Could you check a few things on this model? Use its own coordinates, in mm. A direction names the side the tool comes from. Give positions to 0.01 mm unless a question says otherwise; leave off trailing zeros. Write each loop counter-clockwise with the first axis right and the second up, starting at its lowest first coordinate (ties: lowest second). Pieces come first, ordered by that corner, then holes. Notation, with made-up numbers: M 11.25,63 L 60.25,63 A7 ccw 60.25,74 Z; hole C 63,79 d5. An arc over 180 degrees is marked long. Answer as CSV lines item,"result". Start each with the question number.
Autodesk Inventor part; units mm, degrees
ref_plane "作業平面1" through (0, 0, 29) normal (0, 0, 1) x (1, 0, 0)
ref_plane "YZ Plane" through (0, 0, 0) normal (1, 0, 0) x (0, 1, 0)
ref_plane "XZ Plane" through (0, 0, 0) normal (0, 1, 0) x (-1, 0, 0)
sketch "スケッチ1" plane through (0, 0, 0) normal (0, 0, 1) x (1, 0, 0)
  circle A0 centre (0, 0) radius 1.5
  circle A1 centre (0, 0) radius 3
  dimension "d0" = 3
  dimension "d1" = 6
extrude "押し出し1" add sketch "スケッチ1" along normal blind 35
ref_plane "作業平面1" through (0, 0, 29) normal (0, 0, 1) x (1, 0, 0)
sketch "スケッチ3" plane through (0, 0, 29) normal (0, 0, 1) x (1, 0, 0)
  circle A0 centre (0, 0) radius 1.5
extrude "押し出し3" add sketch "スケッチ3" against normal blind 23
sketch "スケッチ4" plane through (0, 0, 0) normal (0, 0, -1) x (-1, 0, 0)
  circle A0 centre (0, 0) radius 3
  circle A1 centre (0, 0) radius 1.5
  circle A2 centre (0, 0) radius 3
  circle A3 centre (0, 0) radius 4
  dimension "d9" = 8
extrude "押し出し4" add sketch "スケッチ4" against normal blind 35 contours A3
sketch "スケッチ5" plane through (0, 0, 35) normal (0, 0, 1) x (1, 0, 0)
  circle A0 centre (0, 0) radius 1.5
  circle A1 centre (0, 0) radius 2
  dimension "d12" = 4
extrude "押し出し5" cut sketch "スケッチ5" against normal blind 6 contours A0 | A1
properties part number "スペーサー自作m3,35" material "アルミニウム 7075"
1. On a 3-axis mill with a long thin cutter (end or side, diameter ignored), from which of +Z, -Z, +X, -X, +Y, -Y can I reach the whole of each face in a straight line? I mean faces 5 (the flat face through (2, -1, 35)), 6 (the flat face through (0, 0, 29)), 7 (the flat face through (0, 0, 6)). Say none if no direction works.
2. Imagine slicing it at D-D, the plane y = 3.25. Please give me the cut outline in (x, z), plus the area to 3 significant figures.
3. Imagine slicing it at B-B, the plane z = 25.5. Please give me the cut outline in (x, y).
4. Imagine slicing it at C-C, the plane y = -2.75. Please give me the cut outline in (x, z), plus the area to 3 significant figures.
5. Thinking about a two-plate mould opening in X: for faces 1 (the flat face through (-2, 0, 0)), 2 (the cylindrical face through (0.867, -3.905, 17.255)), 3 (the cylindrical face through (-1.5, -0.07, 2.96)), 4 (the cylindrical face through (0, -2, 32)), which applies, pulls with the +X half, pulls with the -X half, needs draft (parallel to the pull), parting line crosses it, or undercut?
6. Please list where these lines run through material, in increasing order: line 1 (Y direction, x = 0, z = 4.05); line 2 (Y direction, x = 0, z = 32.85); line 3 (Z direction, x = -1.75, y = 0).
7. Will these pins go through, and if not, where does the flat tip stop? P1, Ø3, axis at x = -2.5, z = 14.5, coming from the +Y side; P2, Ø1.5, axis at x = 0, y = 0.5, coming from the -Z side; P3, Ø1.2, axis at x = -0.5, y = -0.5, coming from the +Z side.
8. Imagine slicing it at A-A, the plane x = 0. Please give me the cut outline in (y, z), plus the area to 3 significant figures.
Solutions:
1,face 5,"+Z, +X, -X, +Y, -Y"
1,face 6,"+Z"
1,face 7,"-Z"
2,outline,"M -2.33,0 L 2.33,0 L 2.33,35 L -2.33,35 Z"
2,area,"163 mm²"
3,outline,"C 0,0 d8"
4,outline,"M -2.9,0 L 2.9,0 L 2.9,35 L -2.9,35 Z"
4,area,"203 mm²"
5,face 1,"needs draft"
5,face 2,"parting line crosses it"
5,face 3,"undercut"
5,face 4,"undercut"
6,line 1,"-4 to -1.5, 1.5 to 4"
6,line 2,"-4 to -2, 2 to 4"
6,line 3,"0 to 29"
7,P1,"y = 3.87"
7,P2,"z = 6"
7,P3,"z = 29"
8,outline,"M -4,0 L -1.5,0 L -1.5,6 L 1.5,6 L 1.5,0 L 4,0 L 4,35 L 2,35 L 2,29 L -2,29 L -2,35 L -4,35 Z"
8,area,"238 mm²"
